from build123d import *

# Parameters (mm, degrees)
SKETCH1_W             = 50.8
SKETCH1_H             = 25.4
SKETCH1_W_2           = 45.72
SKETCH1_H_2           = 20.32
BOSS_EXTRUDE1_DEPTH   = 533.4
F_8_CLEARANCE_HOLE1_D = 4.4958
CUT_EXTRUDE2_DEPTH    = 76.962
SKETCH5_R             = 14.2875
CUT_EXTRUDE3_DEPTH    = 43.434


with BuildPart() as part:
    # Sketch1 → Boss-Extrude1 (new body)
    with BuildSketch(Plane.XY):
        Rectangle(SKETCH1_W, SKETCH1_H)
        Rectangle(SKETCH1_W_2, SKETCH1_H_2, mode=Mode.SUBTRACT)
    extrude(amount=-BOSS_EXTRUDE1_DEPTH)

    # #8 Clearance Hole1 (through all)
    with Locations(Plane(origin=(25.4, 0, 0), x_dir=(0, 0, -1), z_dir=(1, 0, 0))):
        with Locations((12.7, 0), (38.1, 0), (63.5, 0), (88.9, 0), (114.3, 0), (139.7, 0), (165.1, 0), (190.5, 0), (215.9, 0), (241.3, 0), (266.7, 0), (292.1, 0), (317.5, 0), (342.9, 0), (368.3, 0), (393.7, 0), (419.1, 0), (444.5, 0), (469.9, 0), (495.3, 0), (520.7, 0)):
            Hole(F_8_CLEARANCE_HOLE1_D / 2)

    # Sketch4 → Cut-Extrude2 (cut)
    with BuildSketch(Plane(origin=(0, 12.7, 0), x_dir=(1, 0, 0), z_dir=(0, 1, 0))):
        Polygon((-7.206301081, 228.6), (135.513081356, 228.6), (135.513081356, -17.641370014), (-94.056886123, -17.641370014), (-94.056886123, 228.6), align=None)
    extrude(amount=-CUT_EXTRUDE2_DEPTH, mode=Mode.SUBTRACT)

    # Sketch5 → Cut-Extrude3 (cut)
    with BuildSketch(Plane(origin=(0, 12.7, 0), x_dir=(1, 0, 0), z_dir=(0, 1, 0))):
        with Locations((0, 493.7125)):
            Circle(SKETCH5_R)
        with Locations((0, 303.2125)):
            Circle(SKETCH5_R)
    extrude(amount=-CUT_EXTRUDE3_DEPTH, mode=Mode.SUBTRACT)


solid = part.part
Part model, mm, in its own coordinate system. A direction names the side the tool comes from. Round coordinates to 2 decimals unless told otherwise and drop trailing zeros. Write each loop counter-clockwise with the first axis right and the second up, starting at its lowest first coordinate (ties: lowest second). Pieces come first, ordered by that corner, then holes. Notation, with made-up numbers: (59, 47) - (73, 47) arc R20 cw to (73, 83) - close; hole circle Ø10 at (88, 57.25). An arc over 180 degrees is marked (long way). Use CSV: the item, a comma, the result in double quotes.
Item 1: Tool access for faces 4 (the flat face through (0, 10.16, -379)), 5 (the flat face through (-0.1, 10.4, -533.4)): list every direction of +Z, -Z, +X, -X, +Y, -Y with a clear straight run to the whole face (end or side of a thin tool).
Results list:
face 4,"+Z, -Z"
face 5,"-Z, +X, -X, +Y, -Y"
Item 2: Slice it at D-D, the plane z = -300.5. Write the cut outline in (x, y).
Results list:
outline,"(-25.4, -12.7) - (-14.03, -12.7) - (-14.03, -10.16) - (-22.86, -10.16) - (-22.86, 10.16) - (-14.03, 10.16) - (-14.03, 12.7) - (-25.4, 12.7) - close; (14.03, -12.7) - (25.4, -12.7) - (25.4, 12.7) - (14.03, 12.7) - (14.03, 10.16) - (22.86, 10.16) - (22.86, -10.16) - (14.03, -10.16) - close"
Item 3: Slice it at C-C, the plane z = -450. Write the cut outline in (x, y).
Results list:
outline,"(-25.4, -12.7) - (25.4, -12.7) - (25.4, 12.7) - (-25.4, 12.7) - close; hole (-22.86, -10.16) - (22.86, -10.16) - (22.86, 10.16) - (-22.86, 10.16) - close"
Item 4: Slice it at A-A, the plane y = 5.75. Write the cut outline in (x, z), then the cut area to 3 significant figures.
Results list:
outline,"(-25.4, -533.4) - (-22.86, -533.4) - (-22.86, -228.6) - (-25.4, -228.6) - close; (22.86, -533.4) - (25.4, -533.4) - (25.4, -228.6) - (22.86, -228.6) - close"
area,"1,550 mm²"
Item 5: Slice it at B-B, the plane x = 0. Write the cut outline in (y, z) (3 decimals), then the cut area to 3 significant figures.
Results list:
outline,"(-12.7, -533.4) - (-10.16, -533.4) - (-10.16, -508) - (-12.7, -508) - close; (-12.7, -479.425) - (-10.16, -479.425) - (-10.16, -317.5) - (-12.7, -317.5) - close; (-12.7, -288.925) - (-10.16, -288.925) - (-10.16, -228.6) - (-12.7, -228.6) - close; (10.16, -533.4) - (12.7, -533.4) - (12.7, -508) - (10.16, -508) - close; (10.16, -479.425) - (12.7, -479.425) - (12.7, -317.5) - (10.16, -317.5) - close; (10.16, -288.925) - (12.7, -288.925) - (12.7, -228.6) - (10.16, -228.6) - close"
area,"1,260 mm²"
Item 6: Flat gauge pin, fed straight in: P1, Ø7, axis at y = 0, z = -520.7, coming from the -X side. Where does the tip first touch, or does it go through?
Results list:
P1,"stops at x = -25.4"
Item 7: Wall check: L1, parallel to Z at x = 0, y = -10.7 (3 decimals); L2, parallel to X at y = -9, z = -445; L3, parallel to Y at x = -16.5, z = -424. Give the ranges that are in metal, low to high.
Results list:
L1,"z = -533.4 to -508, -479.425 to -317.5, -288.925 to -228.6"
L2,"x = -25.4 to -22.86, 22.86 to 25.4"
L3,"y = -12.7 to -10.16, 10.16 to 12.7"
Item 8: Pull direction X, two halves, no side cores. Call faces 1 (the flat face through (25.4, 0, -379)), 2 (the cylindrical face through (-3.097, -11.412, -479.765)), 3 (the flat face through (0, -12.7, -379)): pulls with the +X half, pulls with the -X half, needs draft (parallel to the pull), parting line crosses it, or undercut.
Results list:
face 1,"pulls with the +X half"
face 2,"undercut"
face 3,"needs draft"
